```python
from build123d import *

# Parameters (mm, degrees)
SCHIZZO1_W                   = 46
SCHIZZO1_H                   = 44.5
ESTRUSIONE_ESTRUSIONE1_DEPTH = 11
SCHIZZO2_W                   = 23
SCHIZZO2_H                   = 20.5
ESTRUSIONE_ESTRUSIONE2_DEPTH = 2
TAGLIO_ESTRUSIONE1_DEPTH     = 5.5
SCHIZZO5_W                   = 38.5
SCHIZZO5_H                   = 9
TAGLIO_ESTRUSIONE2_DEPTH     = 1
SCHIZZO9_W                   = 10
SCHIZZO9_H                   = 3
TAGLIO_ESTRUSIONE4_DEPTH     = 1
SCHIZZO10_W                  = 5
SCHIZZO10_H                  = 23
TAGLIO_ESTRUSIONE5_DEPTH     = 3
SCHIZZO11_W                  = 5
SCHIZZO11_H                  = 14
TAGLIO_ESTRUSIONE6_DEPTH     = 2
FORO_PER_VITE_M1_2_D         = 1.2
SVUOTA3_OUTLINE_W            = 12
SVUOTA3_OUTLINE_H            = 5
SVUOTA3_DEPTH                = 10
SVUOTA3_2_OUTLINE_W          = 5
SVUOTA3_2_OUTLINE_H          = 25
SVUOTA3_2_OUTLINE_W_2        = 12
SVUOTA3_2_OUTLINE_H_2        = 5
SVUOTA3_2_DEPTH              = 5
SVUOTA3_START                = 10
SVUOTA3_3_OUTLINE_W          = 21
SVUOTA3_3_OUTLINE_H          = 18.5
SVUOTA3_3_DEPTH              = 2
SVUOTA3_START_2              = 5
SVUOTA3_4_OUTLINE_W          = 12
SVUOTA3_4_OUTLINE_H          = 5
SVUOTA3_4_DEPTH              = 4
SVUOTA3_5_OUTLINE_W          = 5
SVUOTA3_5_OUTLINE_H          = 9
SVUOTA3_5_DEPTH              = 2
SVUOTA3_6_DEPTH              = 4.5


# Read off the part's stored shape, not the designer's step: Svuota3
with BuildPart() as part:
    # Schizzo1 → Estrusione-Estrusione1 (new body)
    with BuildSketch(Plane(origin=(0, 0, 0), x_dir=(1, 0, 0), z_dir=(0, 1, 0))):
        Rectangle(SCHIZZO1_W, SCHIZZO1_H)
    extrude(amount=ESTRUSIONE_ESTRUSIONE1_DEPTH)

    # Schizzo2 → Estrusione-Estrusione2 (add)
    with BuildSketch(Plane(origin=(0, 11, 0), x_dir=(1, 0, 0), z_dir=(0, 1, 0))):
        with Locations((6.5, 8.5)):
            Rectangle(SCHIZZO2_W, SCHIZZO2_H)
    extrude(amount=ESTRUSIONE_ESTRUSIONE2_DEPTH)

    # Schizzo3 → Taglio-Estrusione1 (cut)
    with BuildSketch(Plane(origin=(0, 11, 0), x_dir=(1, 0, 0), z_dir=(0, 1, 0))):
        with BuildLine():
            Line((23, 22.25), (20.5, 22.25))
            Line((20.5, 22.25), (20.5, 20.25))
            ThreePointArc((20.5, 20.25), (20.646446609, 19.896446609), (21, 19.75))
            Line((21, 19.75), (23, 19.75))
            Line((23, 19.75), (23, 22.25))
        make_face()
        with BuildLine():
            Line((23, -22.25), (20.5, -22.25))
            Line((20.5, -22.25), (20.5, -20.25))
            ThreePointArc((20.5, -20.25), (20.646446609, -19.896446609), (21, -19.75))
            Line((21, -19.75), (23, -19.75))
            Line((23, -19.75), (23, -22.25))
        make_face()
        with BuildLine():
            Line((-20, 22.25), (-18, 22.25))
            Line((-18, 22.25), (-18, 20.25))
            ThreePointArc((-18, 20.25), (-18.146446609, 19.896446609), (-18.5, 19.75))
            Line((-18.5, 19.75), (-19.5, 19.75))
            ThreePointArc((-19.5, 19.75), (-19.853553391, 19.896446609), (-20, 20.25))
            Line((-20, 20.25), (-20, 22.25))
        make_face()
        with BuildLine():
            Line((-20, -22.25), (-18, -22.25))
            Line((-18, -22.25), (-18, -20.25))
            ThreePointArc((-18, -20.25), (-18.146446609, -19.896446609), (-18.5, -19.75))
            Line((-18.5, -19.75), (-19.5, -19.75))
            ThreePointArc((-19.5, -19.75), (-19.853553391, -19.896446609), (-20, -20.25))
            Line((-20, -20.25), (-20, -22.25))
        make_face()
    extrude(amount=-TAGLIO_ESTRUSIONE1_DEPTH, mode=Mode.SUBTRACT)

    # Schizzo5 → Taglio-Estrusione2 (cut)
    with BuildSketch(Plane(origin=(-23, 0, -0.75), x_dir=(0, 0, -1), z_dir=(1, 0, 0))):
        with Locations((-0.75, 4.5)):
            Rectangle(SCHIZZO5_W, SCHIZZO5_H)
    extrude(amount=TAGLIO_ESTRUSIONE2_DEPTH, mode=Mode.SUBTRACT)

    # Schizzo9 → Taglio-Estrusione4 (cut)
    with BuildSketch(Plane(origin=(0, 11, 0), x_dir=(1, 0, 0), z_dir=(0, 1, 0))):
        with Locations((-13, -0.25)):
            Rectangle(SCHIZZO9_W, SCHIZZO9_H)
    extrude(amount=-TAGLIO_ESTRUSIONE4_DEPTH, mode=Mode.SUBTRACT)

    # Schizzo10 → Taglio-Estrusione5 (cut)
    with BuildSketch(Plane(origin=(0, 11, 0), x_dir=(1, 0, 0), z_dir=(0, 1, 0))):
        with Locations((20.5, -6.25)):
            Rectangle(SCHIZZO10_W, SCHIZZO10_H)
    extrude(amount=-TAGLIO_ESTRUSIONE5_DEPTH, mode=Mode.SUBTRACT)

    # Schizzo11 → Taglio-Estrusione6 (cut)
    with BuildSketch(Plane(origin=(0, 8, 0), x_dir=(1, 0, 0), z_dir=(0, 1, 0))):
        with Locations((20.5, -10.75)):
            Rectangle(SCHIZZO11_W, SCHIZZO11_H)
    extrude(amount=-TAGLIO_ESTRUSIONE6_DEPTH, mode=Mode.SUBTRACT)

    # Foro per Vite M1-2 (through all)
    with Locations(Plane(origin=(0, 5.5, 0), x_dir=(1, 0, 0), z_dir=(0, 1, 0))):
        with Locations((21.34, -20.59), (21.335553897, 20.599331768), (-19, 20.5), (-19, -20.5)):
            Hole(FORO_PER_VITE_M1_2_D / 2)

    # Svuota3 outline → Svuota3 (cut)
    with BuildSketch(Plane(origin=(0, 0, 0), x_dir=(1, 0, 0), z_dir=(0, 1, 0))):
        with BuildLine():
            Line((22, 6.25), (22, 18.75))
            Line((22, 18.75), (21, 18.75))
            ThreePointArc((21, 18.75), (19.939339828, 19.189339828), (19.5, 20.25))
            Line((19.5, 20.25), (19.5, 21.25))
            Line((19.5, 21.25), (-17, 21.25))
            Line((-17, 21.25), (-17, 20.25))
            ThreePointArc((-17, 20.25), (-17.439339828, 19.189339828), (-18.5, 18.75))
            Line((-18.5, 18.75), (-19.5, 18.75))
            ThreePointArc((-19.5, 18.75), (-20.560660172, 19.189339828), (-21, 20.25))
            Line((-21, 20.25), (-21, 21.25))
            Line((-21, 21.25), (-22, 21.25))
            Line((-22, 21.25), (-22, -21.25))
            Line((-22, -21.25), (-21, -21.25))
            Line((-21, -21.25), (-21, -20.25))
            ThreePointArc((-21, -20.25), (-20.560660172, -19.189339828), (-19.5, -18.75))
            Line((-19.5, -18.75), (-18.5, -18.75))
            ThreePointArc((-18.5, -18.75), (-17.439339828, -19.189339828), (-17, -20.25))
            Line((-17, -20.25), (-17, -21.25))
            Line((-17, -21.25), (19.5, -21.25))
            Line((19.5, -21.25), (19.5, -20.25))
            ThreePointArc((19.5, -20.25), (19.939339828, -19.189339828), (21, -18.75))
            Line((21, -18.75), (17, -18.75))
            Line((17, -18.75), (17, 6.25))
            Line((17, 6.25), (22, 6.25))
        make_face()
        with Locations((-13, -0.25)):
            Rectangle(SVUOTA3_OUTLINE_W, SVUOTA3_OUTLINE_H, mode=Mode.SUBTRACT)
    extrude(amount=SVUOTA3_DEPTH, mode=Mode.SUBTRACT)

    # Svuota3 2 outline → Svuota3 2 (cut)
    with BuildSketch(Plane(origin=(0, 0, 0), x_dir=(1, 0, 0), z_dir=(0, 1, 0))):
        with Locations((19.5, -6.25)):
            Rectangle(SVUOTA3_2_OUTLINE_W, SVUOTA3_2_OUTLINE_H)
        with Locations((-13, -0.25)):
            Rectangle(SVUOTA3_2_OUTLINE_W_2, SVUOTA3_2_OUTLINE_H_2)
    extrude(amount=SVUOTA3_2_DEPTH, mode=Mode.SUBTRACT)

    # Svuota3 3 outline → Svuota3 3 (cut)
    with BuildSketch(Plane(origin=(0, 0, 0), x_dir=(1, 0, 0), z_dir=(0, 1, 0)).offset(SVUOTA3_START)):
        with Locations((6.5, 8.5)):
            Rectangle(SVUOTA3_3_OUTLINE_W, SVUOTA3_3_OUTLINE_H)
    extrude(amount=SVUOTA3_3_DEPTH, mode=Mode.SUBTRACT)

    # Svuota3 4 outline → Svuota3 4 (cut)
    with BuildSketch(Plane(origin=(0, 0, 0), x_dir=(1, 0, 0), z_dir=(0, 1, 0)).offset(SVUOTA3_START_2)):
        with Locations((-13, -0.25)):
            Rectangle(SVUOTA3_4_OUTLINE_W, SVUOTA3_4_OUTLINE_H)
    extrude(amount=SVUOTA3_4_DEPTH, mode=Mode.SUBTRACT)

    # Svuota3 5 outline → Svuota3 5 (cut)
    with BuildSketch(Plane(origin=(0, 0, 0), x_dir=(1, 0, 0), z_dir=(0, 1, 0)).offset(SVUOTA3_START_2)):
        with Locations((19.5, 1.75)):
            Rectangle(SVUOTA3_5_OUTLINE_W, SVUOTA3_5_OUTLINE_H)
    extrude(amount=SVUOTA3_5_DEPTH, mode=Mode.SUBTRACT)

    # Svuota3 6 outline → Svuota3 6 (cut)
    with BuildSketch(Plane(origin=(0, 0, 0), x_dir=(1, 0, 0), z_dir=(0, 1, 0))):
        with BuildLine():
            Line((22, 18.75), (22, 19.143821075))
            ThreePointArc((22, 19.143821075), (20.209538985, 19.462630216), (19.873832018, 21.25))
            Line((19.873832018, 21.25), (19.5, 21.25))
            Line((19.5, 21.25), (19.5, 20.25))
            ThreePointArc((19.5, 20.25), (19.939339828, 19.189339828), (21, 18.75))
            Line((21, 18.75), (22, 18.75))
        make_face()
        with BuildLine():
            Line((-17, 20.25), (-17, 21.25))
            Line((-17, 21.25), (-17.586670597, 21.25))
            ThreePointArc((-17.586670597, 21.25), (-19, 18.9), (-20.413329403, 21.25))
            Line((-20.413329403, 21.25), (-21, 21.25))
            Line((-21, 21.25), (-21, 20.25))
            ThreePointArc((-21, 20.25), (-20.560660172, 19.189339828), (-19.5, 18.75))
            Line((-19.5, 18.75), (-18.5, 18.75))
            ThreePointArc((-18.5, 18.75), (-17.439339828, 19.189339828), (-17, 20.25))
        make_face()
        with BuildLine():
            Line((22, -19.132467839), (22, -18.75))
            Line((22, -18.75), (21, -18.75))
            ThreePointArc((21, -18.75), (19.939339828, -19.189339828), (19.5, -20.25))
            Line((19.5, -20.25), (19.5, -21.25))
            Line((19.5, -21.25), (19.882467839, -21.25))
            ThreePointArc((19.882467839, -21.25), (20.20862915, -19.45862915), (22, -19.132467839))
        make_face()
        with BuildLine():
            Line((-17.586670597, -21.25), (-17, -21.25))
            Line((-17, -21.25), (-17, -20.25))
            ThreePointArc((-17, -20.25), (-17.439339828, -19.189339828), (-18.5, -18.75))
            Line((-18.5, -18.75), (-19.5, -18.75))
            ThreePointArc((-19.5, -18.75), (-20.560660172, -19.189339828), (-21, -20.25))
            Line((-21, -20.25), (-21, -21.25))
            Line((-21, -21.25), (-20.413329403, -21.25))
            ThreePointArc((-20.413329403, -21.25), (-19, -18.9), (-17.586670597, -21.25))
        make_face()
    extrude(amount=SVUOTA3_6_DEPTH, mode=Mode.SUBTRACT)


solid = part.part
```
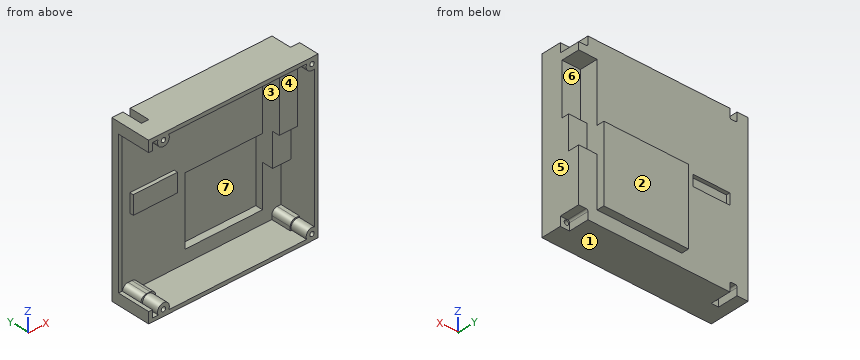
Check sheet for the modelled part. Datum: model origin and axes. Units: mm. Face numbers are marked on the shaded views. A direction names the side the tool comes from. Coordinates: 2 decimals unless noted, no trailing zeros. Loops run counter-clockwise (first coordinate to the right, second up) from the corner with the lowest first, then second, coordinate; pieces in that order, holes last.
1) Sectioned sample at A-A (x = 1). Record the boundary of the cut face in (y, z).
2) Material ranges on probe 1 along X at (y, z) = (4.4, -20.5); probe 2 along Z at (x, y) = (-17, 3.75); probe 3 along Z at (x, y) = (-13, 10.5), recorded low to high.
3) Sectioned sample at B-B (z = -9.5). Record the boundary of the cut face in (x, y), and give its area (3 significant figures).
4) Gauge pin test, flat ends, axial feed: pin 1 (2 mm diameter, centred on x = 17, z = 9.5, fed in from +Y); pin 2 (4 mm diameter, centred on x = 12.5, z = -16.5, fed in from -Y); pin 3 (1.5 mm diameter, centred on x = -10.5, z = 0.5, fed in from -Y). Record the tip position at first contact, or that the pin passes through.
5) Access from +Z, -Z, +X, -X, +Y, -Y to the whole of each face (thin tool, end or side, straight path). Record for the marked faces 4, 5, 6 and 7.
6) Release check for a two-part mould opening along Z. For the marked faces 1, 2 and 3 record: released by +Z, released by -Z, zero draft, split by the parting line, or undercut.
7) Sectioned sample at C-C (y = 3). Record the boundary of the cut face in (x, z), and give its area (3 significant figures).
8) Sectioned sample at D-D (z = 7). Record the boundary of the cut face in (x, y), and give its area (3 significant figures).
Check sheet entries:
1. outline: (0, -22.25) - (11, -22.25) - (11, -18.75) - (13, -18.75) - (13, 1.75) - (11, 1.75) - (11, 22.25) - (0, 22.25) - (0, 21.25) - (10, 21.25) - (10, 0.75) - (12, 0.75) - (12, -17.75) - (10, -17.75) - (10, -21.25) - (0, -21.25) - close
2. probe 1: x = -23 to -22, -20.6 to -19.6, -18.4 to -17.4, 19.74 to 20.74, 21.93 to 23
2. probe 2: z = -22.25 to -21.25, 21.25 to 22.25
2. probe 3: z = -22.25 to -1.25, 1.75 to 22.25
3. outline: (-23, 9) - (-22, 9) - (-22, 10) - (-4, 10) - (-4, 12) - (17, 12) - (17, 10) - (22, 10) - (22, 0) - (23, 0) - (23, 11) - (18, 11) - (18, 13) - (-5, 13) - (-5, 11) - (-23, 11) - close
3. area: 61.0 mm2
4. pin 1: stops at y = 11
4. pin 2: stops at y = 10
4. pin 3: stops at y = 9
5. face 4: -X, -Y
5. face 5: +Z, -Z, +X, +Y, -Y
5. face 6: +X, +Y
5. face 7: -Y
6. face 1: released by -Z
6. face 2: zero draft
6. face 3: undercut
7. outline: (-23, -22.25) - (23, -22.25) - (23, 22.25) - (-23, 22.25) - (-23, 19.25) - (-22, 19.25) - (-22, 21.25) - (-20.41, 21.25) arc R1.6 ccw (long way) to (-17.59, 21.25) - (19.88, 21.25) arc R1.6 ccw to (22, 19.13) - (22, -19.14) arc R1.6 ccw to (19.87, -21.25) - (-17.59, -21.25) arc R1.6 ccw (long way) to (-20.41, -21.25) - (-22, -21.25) - (-22, -19.25) - (-23, -19.25) - close; hole circle Ø1.2 at (-19, -20.5); hole circle Ø1.2 at (-19, 20.5); hole circle Ø1.2 at (21.34, -20.6); hole circle Ø1.2 at (21.34, 20.59)
7. area: 156 mm2
8. outline: (-23, 9) - (-22, 9) - (-22, 10) - (17, 10) - (17, 5) - (22, 5) - (22, 0) - (23, 0) - (23, 6) - (18, 6) - (18, 11) - (-23, 11) - close
8. area: 57.0 mm2
